Here's how the part is built. I have some questions about the finished solid (model axes, mm). Coordinates: 2 decimals unless noted, no trailing zeros. Write each loop counter-clockwise with the first axis right and the second up, starting at its lowest first coordinate (ties: lowest second). Pieces come first, ordered by that corner, then holes. Notation, with made-up numbers: (-39.5, 12) -> (-14.5, 12) arc R17 cw to (-14.5, 40) -> close; hole circle Ø7 at (76.5, 8.25). An arc over 180 degrees is marked (long way). Use a Markdown table: item, result. Add a question column.
Item 1: Imagine slicing it at A-A, the plane x = -19. Write out the boundary of the cut face in (y, z), and give its area (3 significant figures).
Item 2: Imagine slicing it at B-B, the plane y = 26. Write out the boundary of the cut face in (x, z).
Item 3: If I drill on line 1 along Y through (x, z) = (-48, 6.25); line 2 along X through (y, z) = (26.5, 9); line 3 along X through (y, z) = (21, 3), over which ranges is the centre line in solid material (lowest first)? Write a range as from..to.
Item 4: Imagine slicing it at D-D, the plane y = 10. Write out the boundary of the cut face in (x, z).
Item 5: Will these pins go through, and if not, where does the flat tip stop? pin 1 Ø1.6 at (x, z) = (-51, 9) entering from +Y; pin 2 Ø1.5 at (x, z) = (-33.5, 22.5) entering from +Y; pin 3 Ø5.5 at (y, z) = (10.5, 11) entering from -X.
Item 6: Imagine slicing it at C-C, the plane y = 19. Write out the boundary of the cut face in (x, z), and give its area (3 significant figures).
Item 7: If we mould it in two halves opening along X, with no side actions, what happens to faces 1 (the flat face through (-50, 17.5, 12)), 2 (the cylindrical face through (-13.78, -6.64, 12.32)), 3 (the flat face through (-48, -5.5, 12))? For each: pulls with the +X half, pulls with the -X half, needs draft (parallel to the pull), parting line crosses it, or undercut.
```python
from build123d import *

# Parameters (mm, degrees)
F1_DEPTH = 25


# Not quite as in the source:
# - ends of sketch curves that miss each other by under 0.0002 mm in the source are joined


with BuildPart() as f1:
    # F0 (on Top) → F1 (new body)
    with BuildSketch(Plane.XY):
        with BuildLine():
            Line((-18.380952, 17.5), (-13.180955, 17.5))
            ThreePointArc((-13.180955, 17.5), (-12.9688229656, 17.5878709656), (-12.880955, 17.800003))
            Line((-12.880955, 17.800003), (-12.880952, 29.500001))
            ThreePointArc((-12.880952, 29.500001), (-13.7596316564, 31.6213203436), (-15.880952, 32.5))
            Line((-15.880952, 32.5), (-27.580952, 32.5))
            ThreePointArc((-27.580952, 32.5), (-27.7930840344, 32.4121320344), (-27.880952, 32.2))
            Line((-27.880952, 32.2), (-27.880952, 27))
            Line((-27.880952, 27), (-22.880952, 27))
            Line((-22.880952, 27), (-22.880952, 24.267777))
            Line((-22.880952, 24.267777), (-27.148715, 20))
            Line((-27.148715, 20), (-32.361337, 20))
            Line((-32.361337, 20), (-32.880952, 19.7))
            Line((-32.880952, 19.7), (-33.400567, 20))
            Line((-33.400567, 20), (-38.613181, 20))
            Line((-38.613181, 20), (-42.880937, 24.267771))
            Line((-42.880937, 24.267771), (-42.880952, 27))
            Line((-42.880952, 27), (-37.880952, 27))
            Line((-37.880952, 27), (-37.880952, 32.2))
            ThreePointArc((-37.880952, 32.2), (-37.9688199656, 32.4121320344), (-38.180952, 32.5))
            Line((-38.180952, 32.5), (-49.880952, 32.5))
            ThreePointArc((-49.880952, 32.5), (-52.0022723436, 31.6213203436), (-52.880952, 29.5))
            Line((-52.880952, 29.5), (-52.880952, 17.800003))
            ThreePointArc((-52.880952, 17.800003), (-52.7930810344, 17.5878709656), (-52.580949, 17.500003))
            Line((-52.580949, 17.500003), (-47.380937, 17.5))
            Line((-47.380937, 17.5), (-47.380952, 22.5))
            Line((-47.380952, 22.5), (-44.648728, 22.500001))
            Line((-44.648728, 22.500001), (-40.380952, 18.232248))
            Line((-40.380952, 18.232248), (-40.380952, 13.019615))
            Line((-40.380952, 13.019615), (-40.080952, 12.5))
            Line((-40.080952, 12.5), (-40.380952, 11.980385))
            Line((-40.380952, 11.980385), (-40.380952, 6.767753))
            Line((-40.380952, 6.767753), (-44.648721, 2.499994))
            Line((-44.648721, 2.499994), (-47.380937, 2.500006))
            Line((-47.380937, 2.500006), (-47.380952, 7.5))
            Line((-47.380952, 7.5), (-52.580949, 7.5))
            ThreePointArc((-52.580949, 7.5), (-52.7930810344, 7.4121290344), (-52.880949, 7.199997))
            Line((-52.880949, 7.199997), (-52.880952, -4.5))
            ThreePointArc((-52.880952, -4.5), (-52.0022723436, -6.6213203436), (-49.880952, -7.5))
            Line((-49.880952, -7.5), (-38.180955, -7.5))
            ThreePointArc((-38.180955, -7.5), (-37.9688199656, -7.4121320344), (-37.880952, -7.2))
            Line((-37.880952, -7.2), (-37.880952, -2))
            Line((-37.880952, -2), (-42.880952, -2))
            Line((-42.880952, -2), (-42.880952, 0.732224))
            Line((-42.880952, 0.732224), (-38.613182, 5))
            Line((-38.613182, 5), (-33.400567, 5))
            Line((-33.400567, 5), (-32.880952, 5.3))
            Line((-32.880952, 5.3), (-32.361337, 5))
            Line((-32.361337, 5), (-27.148714, 5))
            Line((-27.148714, 5), (-22.880944, 0.732225))
            Line((-22.880944, 0.732225), (-22.880952, -2))
            Line((-22.880952, -2), (-27.880952, -2))
            Line((-27.880952, -2), (-27.880952, -7.2))
            ThreePointArc((-27.880952, -7.2), (-27.7930840344, -7.4121320344), (-27.580952, -7.5))
            Line((-27.580952, -7.5), (-15.880952, -7.5))
            ThreePointArc((-15.880952, -7.5), (-13.7596316564, -6.6213203436), (-12.880952, -4.5))
            Line((-12.880952, -4.5), (-12.880952, 7.199997))
            ThreePointArc((-12.880952, 7.199997), (-12.9688229656, 7.4121290344), (-13.180955, 7.499997))
            Line((-13.180955, 7.499997), (-18.380952, 7.5))
            Line((-18.380952, 7.5), (-18.380952, 2.5))
            Line((-18.380952, 2.5), (-21.113175, 2.499999))
            Line((-21.113175, 2.499999), (-25.380952, 6.76777))
            Line((-25.380952, 6.76777), (-25.380952, 11.980385))
            Line((-25.380952, 11.980385), (-25.680952, 12.5))
            Line((-25.680952, 12.5), (-25.380952, 13.019615))
            Line((-25.380952, 13.019615), (-25.380952, 18.232231))
            Line((-25.380952, 18.232231), (-21.113175, 22.5))
            Line((-21.113175, 22.5), (-18.380952, 22.5))
            Line((-18.380952, 22.5), (-18.380952, 17.5))
        make_face()
        with BuildLine():
            ThreePointArc((-50.880952, -0.5), (-50.5880587812, 0.2071067812), (-49.880952, 0.5))
            Line((-49.880952, 0.5), (-45.880937, 0.5))
            ThreePointArc((-45.880937, 0.5), (-45.1738452188, 0.2071007812), (-44.880952, -0.500006))
            Line((-44.880952, -0.500006), (-44.880952, -4.5))
            ThreePointArc((-44.880952, -4.5), (-45.1738452188, -5.2071067812), (-45.880952, -5.5))
            Line((-45.880952, -5.5), (-49.880952, -5.5))
            ThreePointArc((-49.880952, -5.5), (-50.5880587812, -5.2071067812), (-50.880952, -4.5))
            Line((-50.880952, -4.5), (-50.880952, -0.5))
        make_face(mode=Mode.SUBTRACT)
        with BuildLine():
            Line((-14.880952, -0.499999), (-14.880952, -4.5))
            ThreePointArc((-14.880952, -4.5), (-15.1738452188, -5.2071067812), (-15.880952, -5.5))
            Line((-15.880952, -5.5), (-19.880952, -5.5))
            ThreePointArc((-19.880952, -5.5), (-20.5880587812, -5.2071067812), (-20.880952, -4.5))
            Line((-20.880952, -4.5), (-20.880952, -0.499999))
            ThreePointArc((-20.880952, -0.499999), (-20.5880587812, 0.2071077812), (-19.880952, 0.500001))
            Line((-19.880952, 0.500001), (-15.880952, 0.500001))
            ThreePointArc((-15.880952, 0.500001), (-15.1738452188, 0.2071077812), (-14.880952, -0.499999))
        make_face(mode=Mode.SUBTRACT)
        with BuildLine():
            ThreePointArc((-37.1869759587, 9.4965590288), (-38.130952, 12.5000067994), (-37.186968179, 15.5034521248))
            ThreePointArc((-37.186968179, 15.5034521248), (-37.1632332946, 15.8875474988), (-37.4865620002, 16.0962359962))
            ThreePointArc((-37.4865620002, 16.0962359962), (-38.1843329758, 17.8032195777), (-36.4771934562, 17.1058309956))
            ThreePointArc((-36.4771934562, 17.1058309956), (-36.2684563797, 16.7822649872), (-35.8841472989, 16.8061954442))
            ThreePointArc((-35.8841472989, 16.8061954442), (-32.8808765483, 17.7499999995), (-29.8776329856, 16.8061090207))
            ThreePointArc((-29.8776329856, 16.8061090207), (-29.4930868042, 16.7824504958), (-29.2847080657, 17.1065090027))
            ThreePointArc((-29.2847080657, 17.1065090027), (-27.578165673, 17.8038098657), (-28.2729980022, 16.0962611865))
            ThreePointArc((-28.2729980022, 16.0962611865), (-28.5981729586, 15.8885199872), (-28.5748681009, 15.5033549322))
            ThreePointArc((-28.5748681009, 15.5033549322), (-27.6309520001, 12.5000377259), (-28.5748248894, 9.4967069229))
            ThreePointArc((-28.5748248894, 9.4967069229), (-28.5986102211, 9.1123426938), (-28.2748899919, 8.9037591925))
            ThreePointArc((-28.2748899919, 8.9037591925), (-27.577743326, 7.1966121229), (-29.2847147364, 7.8941890025))
            ThreePointArc((-29.2847147364, 7.8941890025), (-29.493086142, 8.2175661088), (-29.8770772102, 8.1942793139))
            ThreePointArc((-29.8770772102, 8.1942793139), (-32.8797784079, 7.2500001312), (-35.8829017766, 8.1929363205))
            ThreePointArc((-35.8829017766, 8.1929363205), (-36.2677680781, 8.2180997059), (-36.4771928672, 7.8942229943))
            ThreePointArc((-36.4771928672, 7.8942229943), (-38.1841540665, 7.1966015182), (-37.4870140032, 8.9037593199))
            ThreePointArc((-37.4870140032, 8.9037593199), (-37.1633341924, 9.1122631312), (-37.1869759587, 9.4965590288))
        make_face(mode=Mode.SUBTRACT)
        with BuildLine():
            Line((-49.880952, 30.5), (-45.880952, 30.5))
            ThreePointArc((-45.880952, 30.5), (-45.1738452188, 30.2071067812), (-44.880952, 29.5))
            Line((-44.880952, 29.5), (-44.880952, 25.5))
            ThreePointArc((-44.880952, 25.5), (-45.1738452188, 24.7928932188), (-45.880952, 24.5))
            Line((-45.880952, 24.5), (-49.880952, 24.5))
            ThreePointArc((-49.880952, 24.5), (-50.5880587812, 24.7928932188), (-50.880952, 25.5))
            Line((-50.880952, 25.5), (-50.880952, 29.5))
            ThreePointArc((-50.880952, 29.5), (-50.5880587812, 30.2071067812), (-49.880952, 30.5))
        make_face(mode=Mode.SUBTRACT)
        with BuildLine():
            ThreePointArc((-15.880952, 30.5), (-15.1738452188, 30.2071067812), (-14.880952, 29.5))
            Line((-14.880952, 29.5), (-14.880952, 25.5))
            ThreePointArc((-14.880952, 25.5), (-15.1738452188, 24.7928932188), (-15.880952, 24.5))
            Line((-15.880952, 24.5), (-19.880967, 24.5))
            ThreePointArc((-19.880967, 24.5), (-20.5880587812, 24.7928892188), (-20.880952, 25.499996))
            Line((-20.880952, 25.499996), (-20.880952, 29.5))
            ThreePointArc((-20.880952, 29.5), (-20.5880587812, 30.2071067812), (-19.880952, 30.5))
            Line((-19.880952, 30.5), (-15.880952, 30.5))
        make_face(mode=Mode.SUBTRACT)
    extrude(amount=F1_DEPTH)


solid = f1.part
```
Ans:
| question | item | result |
|---|---|---|
| 1 | outline | (-7.5, 0) -> (-5.5, 0) -> (-5.5, 25) -> (-7.5, 25) -> close; (0.5, 0) -> (2.5, 0) -> (2.5, 25) -> (0.5, 25) -> close; (22.5, 0) -> (24.5, 0) -> (24.5, 25) -> (22.5, 25) -> close; (30.5, 0) -> (32.5, 0) -> (32.5, 25) -> (30.5, 25) -> close |
| 1 | area | 200 mm^2 |
| 2 | outline | (-52.88, 0) -> (-50.88, 0) -> (-50.88, 25) -> (-52.88, 25) -> close; (-44.88, 0) -> (-42.88, 0) -> (-42.88, 25) -> (-44.88, 25) -> close; (-22.88, 0) -> (-20.88, 0) -> (-20.88, 25) -> (-22.88, 25) -> close; (-14.88, 0) -> (-12.88, 0) -> (-12.88, 25) -> (-14.88, 25) -> close |
| 3 | line 1 | y = -7.5..-5.5, 0.5..7.5, 17.5..24.5, 30.5..32.5 |
| 3 | line 2 | x = -52.88..-50.88, -44.88..-42.88, -22.88..-20.88, -14.88..-12.88 |
| 3 | line 3 | x = -52.88..-47.38, -43.15..-39.61, -26.15..-22.61, -18.38..-12.88 |
| 4 | outline | (-40.38, 0) -> (-37.5, 0) -> (-37.5, 25) -> (-40.38, 25) -> close; (-28.26, 0) -> (-25.38, 0) -> (-25.38, 25) -> (-28.26, 25) -> close |
| 5 | pin 1 | stops at y = 32.48 |
| 5 | pin 2 | stops at y = 20 |
| 5 | pin 3 | stops at x = -40.38 |
| 6 | outline | (-52.88, 0) -> (-47.38, 0) -> (-47.38, 25) -> (-52.88, 25) -> close; (-41.15, 0) -> (-24.61, 0) -> (-24.61, 25) -> (-41.15, 25) -> close; (-18.38, 0) -> (-12.88, 0) -> (-12.88, 25) -> (-18.38, 25) -> close |
| 6 | area | 688 mm^2 |
| 7 | face 1 | needs draft |
| 7 | face 2 | pulls with the +X half |
| 7 | face 3 | undercut |
